from build123d import *

# Parameters (mm, degrees)
SKETCH_1_R          = 3.5
EXTRUDE_1_DEPTH     = 16
SKETCH_2_R          = 2
EXTRUDE_2_DEPTH     = 25
SKETCH_3_R          = 3
EXTRUDE_3_DEPTH     = 7
CHAMFER_1_SIZE      = 1
SKETCH_4_R          = 1
CUT_EXTRUDE_1_DEPTH = 26.485289875
SKETCH_5_R          = 2
CUT_EXTRUDE_2_DEPTH = 2


with BuildPart() as part:
    # 草圖1 → 填料-伸長1 (new body)
    with BuildSketch(Plane(origin=(0, 0, 0), x_dir=(1, 0, 0), z_dir=(0, 1, 0))):
        with Locations(Location((0, 0, 0), (0, 0, 270))):
            Circle(SKETCH_1_R)
    extrude(amount=EXTRUDE_1_DEPTH)

    # 草圖2 → 填料-伸長2 (add)
    with BuildSketch(Plane(origin=(0, 0, 0), x_dir=(1, 0, 0), z_dir=(0, 1, 0))):
        with Locations(Location((0, 0, 0), (0, 0, 270))):
            Circle(SKETCH_2_R)
    extrude(amount=EXTRUDE_2_DEPTH)

    # 草圖3 → 填料-伸長3 (add)
    with BuildSketch(Plane(origin=(0, 25, 0), x_dir=(1, 0, 0), z_dir=(0, 1, 0))):
        with Locations(Location((0, 0, 0), (0, 0, 270))):
            Circle(SKETCH_3_R)
    extrude(amount=-EXTRUDE_3_DEPTH)

    # 導角1
    chamfer_1_edges = [part.edges().sort_by_distance(p)[0] for p in [
        (0, 25, -3),
    ]]
    chamfer(chamfer_1_edges, length=CHAMFER_1_SIZE)

    # 草圖4 → 除料-伸長1 (cut, through all)
    with BuildSketch(Plane(origin=(0, 25, 0), x_dir=(1, 0, 0), z_dir=(0, 1, 0))):
        with Locations(Location((0, 0, 0), (0, 0, 270))):
            Circle(SKETCH_4_R)
    extrude(amount=-CUT_EXTRUDE_1_DEPTH, mode=Mode.SUBTRACT)

    # 草圖5 → 除料-伸長2 (cut)
    with BuildSketch(Plane(origin=(0, 0, 0), x_dir=(-1, 0, 0), z_dir=(0, -1, 0))):
        with Locations(Location((0, 0, 0), (0, 0, 270))):
            Circle(SKETCH_5_R)
    extrude(amount=-CUT_EXTRUDE_2_DEPTH, mode=Mode.SUBTRACT)


solid = part.part
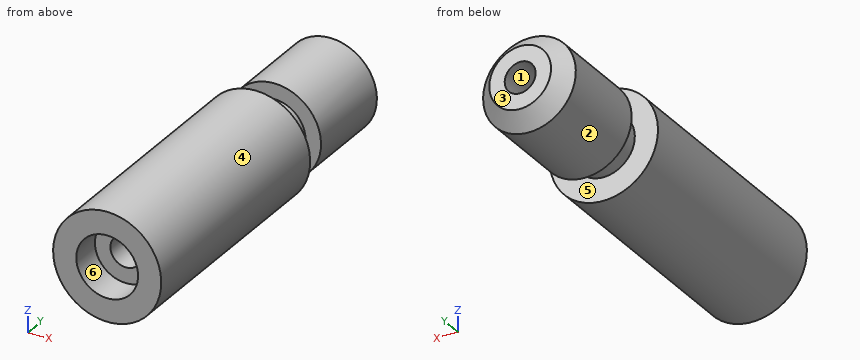
Model file for the job. Use its own axes, mm. Face numbers are marked on the shaded views. A direction names the side the tool comes from. Give positions to 0.01 mm unless a question says otherwise; leave off trailing zeros. Order: outer loops, then holes, each group sorted by start corner. A loop starts at its lowest first (then second) coordinate and runs counter-clockwise, first axis right, second up. Notation, with made-up numbers: (-14.75, 77.25) - (11.25, 77.25) arc R8 cw to (11.25, 83.25) - close; hole circle Ø11 at (-3.5, 20.25). An arc over 180 degrees is marked (long way). Write item = value, one per line. Start each with the question number.
1. Probe line 1 along X through (y, z) = (19.75, 0); line 2 along X through (y, z) = (9.5, 0); line 3 along Z through (x, y) = (0.5, 22.25). List the from-to ranges inside material, lowest first.
2. Two-plate mould, pull along X, no slides. Class the marked faces 1, 2 and 3: pulls with the +X half, pulls with the -X half, needs draft (parallel to the pull), parting line crosses it, or undercut.
3. Cut at C-C, the plane y = 7. List the corners of the cut face in (x, z), and give its area (3 significant figures).
4. Cut at D-D, the plane y = 23.25. List the corners of the cut face in (x, z).
5. Cut at A-A, the plane z = 0. List the corners of the cut face in (x, y).
6. Cut at B-B, the plane x = 0. List the corners of the cut face in (y, z), and give its area (3 significant figures).
7. Which spindle directions (+Z, -Z, +X, -X, +Y, -Y) get a long thin tool onto all of the face, cutting with end or side? Do the marked faces 4, 5 and 6. Say none if no direction does.
8. Drop flat-ended pins along their axis: P1, Ø3, axis at x = 0, z = 0, coming from the +Y side; P2, Ø1.2, axis at x = 0, z = 0, coming from the +Y side. Give the stop position or say it passes through.
Taken from the geometry:
q1.line_1 = -3 to -1, 1 to 3
q1.line_2 = -3.5 to -1, 1 to 3.5
q1.line_3 = -2.96 to -0.87, 0.87 to 2.96
q2.face_1 = undercut
q2.face_2 = parting line crosses it
q2.face_3 = needs draft
q3.outline = circle Ø7 at (0, 0); hole circle Ø2 at (0, 0)
q3.area = 35.3 mm²
q4.outline = circle Ø6 at (0, 0); hole circle Ø2 at (0, 0)
q5.outline = (-3.5, 0) - (-2, 0) - (-2, 2) - (-1, 2) - (-1, 25) - (-2, 25) - (-3, 24) - (-3, 18) - (-2, 18) - (-2, 16) - (-3.5, 16) - close; (1, 2) - (2, 2) - (2, 0) - (3.5, 0) - (3.5, 16) - (2, 16) - (2, 18) - (3, 18) - (3, 24) - (2, 25) - (1, 25) - close
q6.outline = (0, -3.5) - (16, -3.5) - (16, -2) - (18, -2) - (18, -3) - (24, -3) - (25, -2) - (25, -1) - (2, -1) - (2, -2) - (0, -2) - close; (0, 2) - (2, 2) - (2, 1) - (25, 1) - (25, 2) - (24, 3) - (18, 3) - (18, 2) - (16, 2) - (16, 3.5) - (0, 3.5) - close
q6.area = 107 mm²
q7.face_4 = +Y, -Y
q7.face_5 = none
q7.face_6 = -Y
q8.P1 = 25
q8.P2 = through
